Could you check a few things on this model? Use its own coordinates, in mm. Face numbers are marked on the shaded views. Coordinates: 2 decimals unless noted, no trailing zeros. Loops run counter-clockwise (first coordinate to the right, second up) from the corner with the lowest first, then second, coordinate; pieces in that order, holes last. Notation, with made-up numbers: (35.5, 71.5) - (45.5, 71.5) arc R28 cw to (45.5, 96.5) - close; hole circle Ø10 at (-23.5, 2.25). An arc over 180 degrees is marked (long way). Use CSV: the item, a comma, the result in double quotes.
from build123d import *

# Parameters (mm, degrees)
F0_W     = 800
F0_H     = 440
F1_DEPTH = 9
F3_DEPTH = 40
F4_W     = 50.8
F4_H     = 440
F5_DEPTH = 6
F7_D     = 6


with BuildPart() as f1:
    # F0 (on Top) → F1 (new body, symmetric)
    with BuildSketch(Plane.XY):
        with Locations((0, 220)):
            Rectangle(F0_W, F0_H)
    extrude(amount=F1_DEPTH, both=True)

    # F2 (on face) → F3 (cut)
    with BuildSketch(Plane.XY.offset(9)):
        Polygon((-400, 0), (-100, 0), (-150, 440), (-400, 440), align=None)
        Polygon((150, 440), (100, 0), (400, 0), (400, 440), align=None)
    extrude(amount=-F3_DEPTH, mode=Mode.SUBTRACT)

    # F4 (on face) → F5 (cut)
    with BuildSketch(Plane.XY.offset(9)):
        with Locations((0, 220)):
            Rectangle(F4_W, F4_H)
    extrude(amount=-F5_DEPTH, mode=Mode.SUBTRACT)

    # F7 (through all)
    with Locations(Plane.XY.offset(3)):
        with Locations((-10.4, 430), (10.4, 430), (10.4, 50), (-10.4, 50)):
            Hole(F7_D / 2)


solid = f1.part
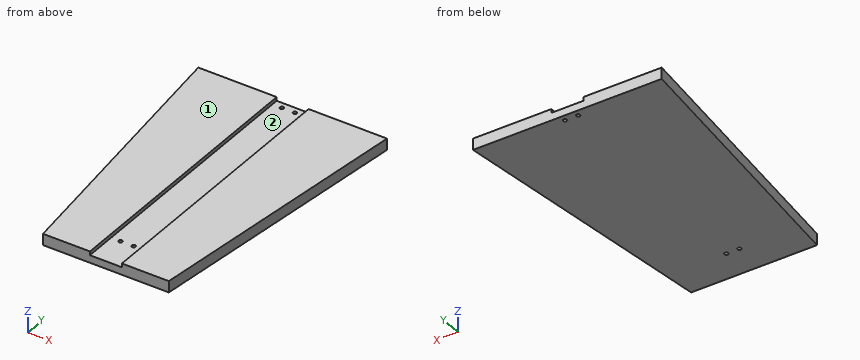
(1) Suppose I cut it at B-B (y = 101). Write out the boundary of the cut face in (x, z), plus the area to 3 significant figures.
Computed:
outline,"(-111.48, -9) - (111.48, -9) - (111.48, 9) - (25.4, 9) - (25.4, 3) - (-25.4, 3) - (-25.4, 9) - (-111.48, 9) - close"
area,"3,710 mm²"
(2) Suppose I cut it at D-D (y = 255). Write out the boundary of the cut face in (x, z), plus the area to 3 significant figures.
Computed:
outline,"(-128.98, -9) - (128.98, -9) - (128.98, 9) - (25.4, 9) - (25.4, 3) - (-25.4, 3) - (-25.4, 9) - (-128.98, 9) - close"
area,"4,340 mm²"
(3) Thinking about a two-plate mould opening in X: for the marked faces 1 and 2, which applies, +X half, -X half, draft (parallel to the pull), parting line (faces both ways), or undercut?
Computed:
face 1,"draft"
face 2,"undercut"
(4) Please list where these lines run through material, in increasing order: line 1 (Y direction, x = 10.4, z = -1.75); line 2 (X direction, y = 430, z = -2); line 3 (X direction, y = 283, z = 7.25).
Computed:
line 1,"y = 0 to 47, 53 to 427, 433 to 440"
line 2,"x = -148.86 to -13.4, -7.4 to 7.4, 13.4 to 148.86"
line 3,"x = -132.16 to -25.4, 25.4 to 132.16"
(5) Will these pins go through, and if not, where does the flat tip stop? pin 1 (2 mm diameter, centred on y = 51.5, z = -1.5, fed in from -X); pin 2 (1.5 mm diameter, centred on y = 320, z = -7, fed in from -X); pin 3 (1 mm diameter, centred on y = 67, z = 5, fed in from +X).
Computed:
pin 1,"stops at x = -105.97"
pin 2,"stops at x = -136.45"
pin 3,"stops at x = 107.67"
(6) Suppose I cut it at C-C (x = 112.5). Write out the boundary of the cut face in (y, z), plus the area to 3 significant figures.
Computed:
outline,"(110, -9) - (440, -9) - (440, 9) - (110, 9) - close"
area,"5,940 mm²"
(7) Suppose I cut it at A-A (z = -4). Write out the boundary of the cut face in (x, y), plus the area to 3 significant figures.
Computed:
outline,"(-150, 440) - (-100, 0) - (100, 0) - (150, 440) - close; hole circle Ø6 at (-10.4, 50); hole circle Ø6 at (-10.4, 430); hole circle Ø6 at (10.4, 50); hole circle Ø6 at (10.4, 430)"
area,"110,000 mm²"
